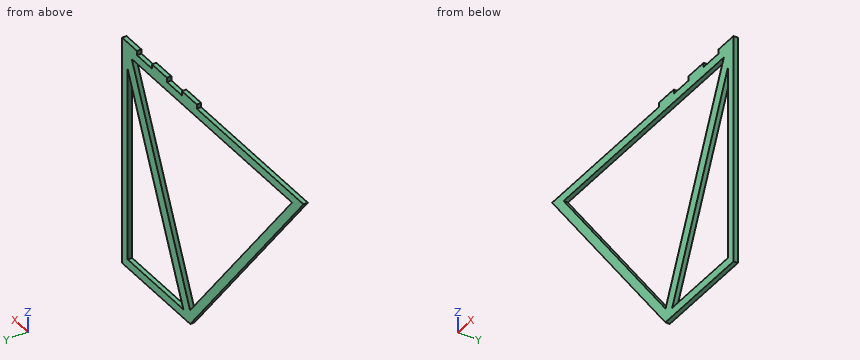
from build123d import *

# Parameters (mm, degrees)
BOSS_EXTRUDE1_DEPTH = 4.7625


with BuildPart() as part:
    # Sketch1 → Boss-Extrude1 (new body)
    with BuildSketch(Plane(origin=(0, 0, 0), x_dir=(1, 0, 0), z_dir=(0, 1, 0))):
        Polygon((-19.475189916, -9.525), (161.925, -9.525), (161.925, -14.2875), (187.325, -14.2875), (187.325, -9.525), (212.725, -9.525), (212.725, -14.2875), (238.125, -14.2875), (238.125, -9.525), (263.525, -9.525), (263.525, -14.2875), (288.925, -14.2875), (288.925, 238.125), (173.141476751, 238.125), align=None)
        Polygon((272.451083662, 0), (0, 0), (173.37796233, 222.914522996), align=None, mode=Mode.SUBTRACT)
        Polygon((184.748916338, 228.6), (279.4, 228.6), (279.4, 15.63506176), align=None, mode=Mode.SUBTRACT)
    extrude(amount=BOSS_EXTRUDE1_DEPTH)


solid = part.part
Design review of the part built by this model. Coordinates are the model's own, in mm. Give positions to 0.01 mm unless a question says otherwise; leave off trailing zeros. Order: outer loops, then holes, each group sorted by start corner. A loop starts at its lowest first (then second) coordinate and runs counter-clockwise, first axis right, second up. Notation, with made-up numbers: (66, -37) - (103, -37) arc R16 ccw to (103, -8) - close; hole circle Ø10 at (-34, 74). An arc over 180 degrees is marked (long way). Use CSV: the item, a comma, the result in double quotes. Start each with the question number.
Q1. For line 1 (X direction, y = 2.2, z = -164.5) (3 decimals); line 2 (X direction, y = 3.5, z = -204) (3 decimals); line 3 (Z direction, x = 214.5, y = 1.3) (1 decimal), list the stretches that pass through material, from the lowest coordinate up.
Q2. Take a section at C-C (z = -103.5). State the section outline as (x, y) points (1 decimal).
Q3. For P1, Ø1.4, axis at x = 249.5, y = 3.5, coming from the +Z side (3 decimals); P2, Ø2, axis at y = 3.5, z = -35.5, coming from the -X side; P3, Ø1.4, axis at y = 3.5, z = 11.5, coming from the -X side (3 decimals), all flat-tipped, find the tip position at first contact; note any pin that passes through.
Q4. Take a section at A-A (y = 3.1). State the section outline as (x, z) points (1 decimal).
Q5. Take a section at D-D (x = 25.5). State the section outline as (y, z) points (1 decimal), and give its area (3 significant figures).
Q6. Take a section at B-B (x = 208.5). State the section outline as (y, z) points (1 decimal), and give its area (3 significant figures).
Calculated:
1,line 1,"x = 115.878 to 127.944, 199.34 to 213.238, 279.4 to 288.925"
1,line 2,"x = 146.6 to 158.667, 181.784 to 195.682, 279.4 to 288.925"
1,line 3,"z = -238.1 to -228.6, -161.7 to -130.4, 0 to 14.3"
2,outline,"(68.4, 0) - (80.5, 0) - (80.5, 4.8) - (68.4, 4.8) - close; (226.5, 0) - (240.3, 0) - (240.3, 4.8) - (226.5, 4.8) - close; (279.4, 0) - (288.9, 0) - (288.9, 4.8) - (279.4, 4.8) - close"
3,P1,"stops at z = 9.525"
3,P2,"stops at x = 14.77"
3,P3,"stops at x = 161.925"
4,outline,"(-19.5, 9.5) - (173.1, -238.1) - (288.9, -238.1) - (288.9, 14.3) - (263.5, 14.3) - (263.5, 9.5) - (238.1, 9.5) - (238.1, 14.3) - (212.7, 14.3) - (212.7, 9.5) - (187.3, 9.5) - (187.3, 14.3) - (161.9, 14.3) - (161.9, 9.5) - close; hole (0, 0) - (173.4, -222.9) - (272.5, 0) - close; hole (184.7, -228.6) - (279.4, -228.6) - (279.4, -15.6) - close"
5,outline,"(0, -48.3) - (4.8, -48.3) - (4.8, -32.8) - (0, -32.8) - close; (0, 0) - (4.8, 0) - (4.8, 9.5) - (0, 9.5) - close"
5,area,"119 mm²"
6,outline,"(0, -238.1) - (4.8, -238.1) - (4.8, -228.6) - (0, -228.6) - close; (0, -175.2) - (4.8, -175.2) - (4.8, -143.9) - (0, -143.9) - close; (0, 0) - (4.8, 0) - (4.8, 9.5) - (0, 9.5) - close"
6,area,"240 mm²"
